Model file for the job. Use its own axes, mm. Face numbers are marked on the shaded views. A direction names the side the tool comes from. Give positions to 0.01 mm unless a question says otherwise; leave off trailing zeros. Loops run counter-clockwise (first coordinate to the right, second up) from the corner with the lowest first, then second, coordinate; pieces in that order, holes last. Notation, with made-up numbers: M 54,89.5 L 103,89.5 A22 cw 103,115.5 Z; hole C 84.5,-17.5 d6. An arc over 180 degrees is marked long. Answer in a Markdown table with one row per item.
```python
from build123d import *

# Parameters (mm, degrees)
BOSS_EXTRU_1_DEPTH      = 5
BOSS_EXTRU_2_DEPTH      = 45
BOSS_EXTRU_3_DEPTH      = 5
ENL_V_MAT_EXTRU_1_REACH = 60.268
ESQUISSE4_R             = 2.75
ENL_V_MAT_EXTRU_2_REACH = 60.631
ESQUISSE5_R             = 2.75


with BuildPart() as part:
    # Esquisse1 → Boss.-Extru.1 (new body)
    with BuildSketch(Plane.XY):
        Polygon((-13.694471154, 7.95), (6.305528846, -12.05), (-13.694471154, -12.05), align=None)
    extrude(amount=BOSS_EXTRU_1_DEPTH)

    # Esquisse2 → Boss.-Extru.2 (add)
    with BuildSketch(Plane.XY.offset(5)):
        Polygon((-13.694471154, -12.05), (6.305528846, -12.05), (1.305528846, -7.05), (-8.694471154, -7.05), (-8.694471154, 2.95), (-13.694471154, 7.95), align=None)
    extrude(amount=BOSS_EXTRU_2_DEPTH)

    # Esquisse3 → Boss.-Extru.3 (add)
    with BuildSketch(Plane.XY.offset(50)):
        Polygon((-13.694471154, 7.95), (6.305528846, -12.05), (-13.694471154, -12.05), align=None)
    extrude(amount=BOSS_EXTRU_3_DEPTH)

    # Esquisse4 → Enlèv. mat.-Extru.1 (cut, up to next)
    with BuildSketch(Plane(origin=(-8.694471154, 0, 0), x_dir=(0, 0, -1), z_dir=(1, 0, 0)), mode=Mode.PRIVATE) as enl_v_mat_extru_1_sk1:
        with Locations((-17.5, -2.05)):
            Circle(ESQUISSE4_R)
    enl_v_mat_extru_1_tool1 = extrude(enl_v_mat_extru_1_sk1.sketch, amount=-ENL_V_MAT_EXTRU_1_REACH, mode=Mode.PRIVATE) & part.part
    # Esquisse4 → Enlèv. mat.-Extru.1 (cut, up to next)
    with BuildSketch(Plane(origin=(-8.694471154, 0, 0), x_dir=(0, 0, -1), z_dir=(1, 0, 0)), mode=Mode.PRIVATE) as enl_v_mat_extru_1_sk2:
        with Locations((-37.5, -2.05)):
            Circle(ESQUISSE4_R)
    enl_v_mat_extru_1_tool2 = extrude(enl_v_mat_extru_1_sk2.sketch, amount=-ENL_V_MAT_EXTRU_1_REACH, mode=Mode.PRIVATE) & part.part
    add(enl_v_mat_extru_1_tool1.solids().sort_by_distance((-8.694471, -2.05, 17.5))[0], mode=Mode.SUBTRACT)
    add(enl_v_mat_extru_1_tool2.solids().sort_by_distance((-8.694471, -2.05, 37.5))[0], mode=Mode.SUBTRACT)

    # Esquisse5 → Enlèv. mat.-Extru.2 (cut, up to next)
    with BuildSketch(Plane(origin=(0, -7.05, 0), x_dir=(1, 0, 0), z_dir=(0, 1, 0)), mode=Mode.PRIVATE) as enl_v_mat_extru_2_sk1:
        with Locations(Location((-3.694471154, -45, 0), (0, 0, 180))):
            Circle(ESQUISSE5_R)
    enl_v_mat_extru_2_tool1 = extrude(enl_v_mat_extru_2_sk1.sketch, amount=-ENL_V_MAT_EXTRU_2_REACH, mode=Mode.PRIVATE) & part.part
    # Esquisse5 → Enlèv. mat.-Extru.2 (cut, up to next)
    with BuildSketch(Plane(origin=(0, -7.05, 0), x_dir=(1, 0, 0), z_dir=(0, 1, 0)), mode=Mode.PRIVATE) as enl_v_mat_extru_2_sk2:
        with Locations(Location((-3.694471154, -27.5, 0), (0, 0, 180))):
            Circle(ESQUISSE5_R)
    enl_v_mat_extru_2_tool2 = extrude(enl_v_mat_extru_2_sk2.sketch, amount=-ENL_V_MAT_EXTRU_2_REACH, mode=Mode.PRIVATE) & part.part
    # Esquisse5 → Enlèv. mat.-Extru.2 (cut, up to next)
    with BuildSketch(Plane(origin=(0, -7.05, 0), x_dir=(1, 0, 0), z_dir=(0, 1, 0)), mode=Mode.PRIVATE) as enl_v_mat_extru_2_sk3:
        with Locations(Location((-3.694471154, -10, 0), (0, 0, 180))):
            Circle(ESQUISSE5_R)
    enl_v_mat_extru_2_tool3 = extrude(enl_v_mat_extru_2_sk3.sketch, amount=-ENL_V_MAT_EXTRU_2_REACH, mode=Mode.PRIVATE) & part.part
    add(enl_v_mat_extru_2_tool1.solids().sort_by_distance((-3.694471, -7.05, 45))[0], mode=Mode.SUBTRACT)
    add(enl_v_mat_extru_2_tool2.solids().sort_by_distance((-3.694471, -7.05, 27.5))[0], mode=Mode.SUBTRACT)
    add(enl_v_mat_extru_2_tool3.solids().sort_by_distance((-3.694471, -7.05, 10))[0], mode=Mode.SUBTRACT)


solid = part.part
```
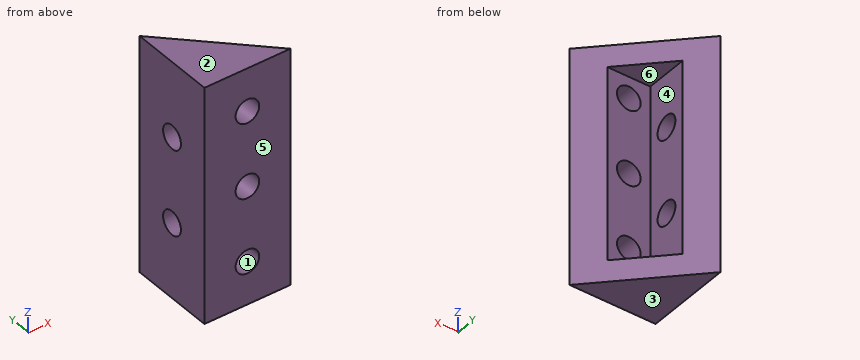
(1) Saw through at C-C, the plane y = -2.05. Give the cut face in (x, z).
Established:
| item | result |
|---|---|
| outline | M -13.69,0 L -3.69,0 L -3.69,5 L -8.69,5 L -8.69,14.75 L -13.69,14.75 Z; M -13.69,20.25 L -8.69,20.25 L -8.69,34.75 L -13.69,34.75 Z; M -13.69,40.25 L -8.69,40.25 L -8.69,50 L -3.69,50 L -3.69,55 L -13.69,55 Z |
(2) Mould opens along Z. For the marked faces 1, 2, 3 and 4 say: pulls with the +Z half, pulls with the -Z half, needs draft (parallel to the pull), parting line crosses it, or undercut.
Established:
| item | result |
|---|---|
| face 1 | undercut |
| face 2 | pulls with the +Z half |
| face 3 | pulls with the -Z half |
| face 4 | undercut |
(3) Saw through at A-A, the plane z = 17.5. Give the cut face in (x, y), and give its area (4 significant figures).
Established:
| item | result |
|---|---|
| outline | M -13.69,-12.05 L 6.31,-12.05 L 1.31,-7.05 L -8.69,-7.05 L -8.69,-4.8 L -13.69,-4.8 Z; M -13.69,0.7 L -8.69,0.7 L -8.69,2.95 L -13.69,7.95 Z |
| area | 122.5 mm2 |
(4) Flat gauge pins, fed straight in: P1, Ø6.5, axis at x = -3.69, z = 27.5, coming from the +Y side; P2, Ø2, axis at y = 5, z = 44, coming from the +X side; P3, Ø11, axis at y = -1, z = 27, coming from the +X side. Where does each tip first touch, or does it go through?
Established:
| item | result |
|---|---|
| P1 | stops at y = -7.05 |
| P2 | stops at x = -9.74 |
| P3 | stops at x = -8.69 |
(5) Saw through at D-D, the plane z = 4. Give the cut face in (x, y).
Established:
| item | result |
|---|---|
| outline | M -13.69,-12.05 L 6.31,-12.05 L -13.69,7.95 Z |
(6) Wall check: L1, parallel to Z at x = -5.5, y = -3; L2, parallel to X at y = -3, z = 12; L3, parallel to Y at x = -5.5, z = 31.5. Give the ranges that are in metal, low to high.
Established:
| item | result |
|---|---|
| L1 | z = 0 to 5, 50 to 55 |
| L2 | x = -13.69 to -8.69 |
| L3 | y = -12.05 to -7.05 |
(7) Saw through at B-B, the plane x = -4.5. Give the cut face in (y, z).
Established:
| item | result |
|---|---|
| outline | M -12.05,0 L -1.24,0 L -1.24,5 L -7.05,5 L -7.05,7.37 L -12.05,7.37 Z; M -12.05,12.63 L -7.05,12.63 L -7.05,24.87 L -12.05,24.87 Z; M -12.05,30.13 L -7.05,30.13 L -7.05,42.37 L -12.05,42.37 Z; M -12.05,47.63 L -7.05,47.63 L -7.05,50 L -1.24,50 L -1.24,55 L -12.05,55 Z |
(8) Which spindle directions (+Z, -Z, +X, -X, +Y, -Y) get a long thin tool onto all of the face, cutting with end or side? Do the marked faces 5 and 6. Say none if no direction does.
Established:
| item | result |
|---|---|
| face 5 | +Z, -Z, +X, -X, -Y |
| face 6 | +X, +Y |
